Geometry check sheet. Reference: the model listing, model coordinates, mm. A direction names the side the tool comes from. Round coordinates to 2 decimals unless told otherwise and drop trailing zeros. Write each loop counter-clockwise with the first axis right and the second up, starting at its lowest first coordinate (ties: lowest second). Pieces come first, ordered by that corner, then holes.
Item 1: Draft check along X on faces 1 (the face through (0, 0, 0)), 2 (the face through (0, -1, -25)), 3 (the face through (2.5, 103, 0)). Enter one of: pulls with the +X half, pulls with the -X half, needs draft (parallel to the pull), parting line crosses it, or undercut.
Item 2: Depth check by flat-ended pin: P1, Ø5, axis at y = 51.5, z = 4.5, coming from the -X side; P2, Ø1, axis at x = 1, y = 64.5, coming from the +Z side; P3, Ø2, axis at y = 104, z = 0, coming from the -X side. Enter the tip coordinate at first touch or a pass-through.
Item 3: Scan lines: probe 1 along Z at (x, y) = (17.5, -0.5); probe 2 along Z at (x, y) = (-17, -1). Record each from-to range of solid material in increasing order.
Item 4: Cross-section at C-C (y = 39.5). Enter the section's corners in (x, z), then the cut area to 3 significant figures.
Item 5: Access from +Z, -Z, +X, -X, +Y, -Y to the whole of each face (thin tool, end or side, straight path). Record for faces 4 (the face through (0, 100, 0)), 5 (the face through (0, 103, 1)), 6 (the face through (-4.88, 50.53, -1.08)), 7 (the face through (0, 103, -1)), 8 (the face through (-1.13, -1.27, -19.27)).
Item 6: Cross-section at A-A (x = -17.5). Enter the section's corners in (y, z).
Item 7: Cross-section at D-D (z = -11). Enter the section's corners in (x, y).
Item 8: Cross-section at B-B (z = -17.5). Enter the section's corners in (x, y).
from build123d import *

# Parameters (mm, degrees)
SKETCH1_R                 = 5
SKETCH1_R_2               = 4.5
BOSS_EXTRUDE1_DEPTH       = 100
SKETCH2_R                 = 5
BOSS_EXTRUDE2_DEPTH       = 2.5
SKETCH3_W                 = 50
SKETCH3_H                 = 50
BOSS_EXTRUDE3_DEPTH       = 2.5
M5X0_8_TAPPED_HOLE1_D     = 4.2
M5X0_8_TAPPED_HOLE1_DEPTH = 14
M5X0_8_TAPPED_HOLE1_TIP   = 1.2618073
SKETCH6_W                 = 5
SKETCH6_H                 = 2
BOSS_EXTRUDE5_DEPTH       = 2


with BuildPart() as part:
    # Sketch1 → Boss-Extrude1 (new body)
    with BuildSketch(Plane(origin=(0, 0, 0), x_dir=(1, 0, 0), z_dir=(0, 1, 0))):
        with Locations(Location((0, 0, 0), (0, 0, 270))):
            Circle(SKETCH1_R)
        with Locations(Location((0, 0, 0), (0, 0, 270))):
            Circle(SKETCH1_R_2, mode=Mode.SUBTRACT)
    extrude(amount=BOSS_EXTRUDE1_DEPTH)

    # Sketch2 → Boss-Extrude2 (add)
    with BuildSketch(Plane(origin=(0, 100, 0), x_dir=(1, 0, 0), z_dir=(0, 1, 0))):
        with Locations(Location((0, 0, 0), (0, 0, 270))):
            Circle(SKETCH2_R)
    extrude(amount=BOSS_EXTRUDE2_DEPTH)

    # Sketch3 → Boss-Extrude3 (add)
    with BuildSketch(Plane.XZ):
        Rectangle(SKETCH3_W, SKETCH3_H)
    extrude(amount=BOSS_EXTRUDE3_DEPTH)

    # M5x0.8 Tapped Hole1
    with Locations(Plane(origin=(0, 0, 0), x_dir=(1, 0, 0), z_dir=(0, 1, 0))):
        with Locations((-17.5, 0), (-17.5, -17.5), (0, -17.5), (17.5, -17.5), (17.5, 0), (17.5, 17.5), (0, 17.5), (-17.5, 17.5)):
            Hole(M5X0_8_TAPPED_HOLE1_D / 2, depth=M5X0_8_TAPPED_HOLE1_DEPTH)
            with Locations((0, 0, -(M5X0_8_TAPPED_HOLE1_DEPTH + M5X0_8_TAPPED_HOLE1_TIP / 2))):  # 118° drill point
                Cone(0, M5X0_8_TAPPED_HOLE1_D / 2, M5X0_8_TAPPED_HOLE1_TIP, mode=Mode.SUBTRACT)

    # Sketch6 → Boss-Extrude5 (add)
    with BuildSketch(Plane(origin=(0, 102.5, 0), x_dir=(1, 0, 0), z_dir=(0, 1, 0))):
        Rectangle(SKETCH6_W, SKETCH6_H)
    extrude(amount=BOSS_EXTRUDE5_DEPTH)


solid = part.part
Resolved:
1. face 1: undercut
1. face 2: needs draft
1. face 3: pulls with the +X half
2. P1: stops at x = -4.58
2. P2: stops at z = 4.97
2. P3: stops at x = -2.5
3. probe 1: z = -25 to -19.6, -15.4 to -2.1, 2.1 to 15.4, 19.6 to 25
3. probe 2: z = -25 to -19.54, -15.46 to -2.04, 2.04 to 15.46, 19.54 to 25
4. outline: circle Ø10 at (0, 0); hole circle Ø9 at (0, 0)
4. area: 14.9 mm2
5. face 4: none
5. face 5: +Z, +X, -X, +Y
5. face 6: +Y
5. face 7: -Z, +X, -X, +Y
5. face 8: +Y, -Y
6. outline: (-2.5, -25) - (0, -25) - (0, -19.6) - (-2.5, -19.6) - close; (-2.5, -15.4) - (0, -15.4) - (0, -2.1) - (-2.5, -2.1) - close; (-2.5, 2.1) - (0, 2.1) - (0, 15.4) - (-2.5, 15.4) - close; (-2.5, 19.6) - (0, 19.6) - (0, 25) - (-2.5, 25) - close
7. outline: (-25, -2.5) - (25, -2.5) - (25, 0) - (-25, 0) - close
8. outline: (-25, -2.5) - (-19.6, -2.5) - (-19.6, 0) - (-25, 0) - close; (-15.4, -2.5) - (-2.1, -2.5) - (-2.1, 0) - (-15.4, 0) - close; (2.1, -2.5) - (15.4, -2.5) - (15.4, 0) - (2.1, 0) - close; (19.6, -2.5) - (25, -2.5) - (25, 0) - (19.6, 0) - close
